Source: CAD feature listing. Evaluate the final solid. Frame: model axes, mm. A direction names the side the tool comes from. Coordinates: 2 decimals unless noted, no trailing zeros. Order: outer loops, then holes, each group sorted by start corner. A loop starts at its lowest first (then second) coordinate and runs counter-clockwise, first axis right, second up. Notation, with made-up numbers: (-12, 51) -> (25, 51) arc R16 cw to (25, 64) -> close; hole circle Ø3 at (38, -38). An arc over 180 degrees is marked (long way). Write item = value, one per line. Start each with the question number.
Item 1: Ray query, line 1 along X through (y, z) = (2.25, 25); line 2 along Z through (x, y) = (12.5, 2.8). Return the intervals inside material, ascending. Write a range as [from, to].
Item 2: Mould query, pull axis X, two halves, no side actions, for faces 3 (the flat face through (-25, 4.5, 14)), 4 (the flat face through (0, 5, 31)), 5 (the cylindrical face through (-14.9, 23.2, 2.5)). Classes: released by +X, released by -X, zero draft, split by the parting line, or undercut.
Item 3: Section query A-A (x = -12.5). Output: boundary loops of the cut face in (y, z), then the cut area to 3 significant figures.
Item 4: Section query B-B (y = 25). Output: boundary loops of the cut face in (x, z).
Item 5: Set-up query: faces 1 (the flat face through (0, 31, 5)), 2 (the flat face through (0, 0, 25)). Return all of +Z, -Z, +X, -X, +Y, -Y with unobstructed straight access to the full face (end or side cutting, diameter ignored); none if empty.
Item 6: Contact query for flat-ended pins moving along their axis: pin 1 (3.5 mm diameter, centred on x = -12.5, z = 25, fed in from -Y); pin 2 (1 mm diameter, centred on x = -1.5, y = 40.5, fed in from +Z); pin 3 (1.5 mm diameter, centred on x = -19.5, z = 17.5, fed in from +Y). Output: stop coordinate, or through.
Item 7: Section query D-D (x = 22.5). Output: boundary loops of the cut face in (y, z).
Autodesk Inventor part; units mm, degrees
ref_plane "YZ Plane" through (0, 0, 0) normal (1, 0, 0) x (0, 1, 0)
ref_plane "XZ Plane" through (0, 0, 0) normal (0, 1, 0) x (-1, 0, 0)
ref_plane "XY Plane" through (0, 0, 0) normal (0, 0, 1) x (1, 0, 0)
sketch "Sketch1" plane through (0, 0, 0) normal (1, 0, 0) x (0, 1, 0)
  line L0 (0, 0) -> (5, 0)
  line L1 (5, 0) -> (5, 50)
  line L2 (5, 50) -> (0, 50)
  line L3 (0, 50) -> (0, 0)
  line L4 (0, 0) -> (50, 0)
  line L5 (50, 0) -> (50, 5)
  line L6 (50, 5) -> (0, 5)
  line L7 (0, 5) -> (0, 0)
  point P0 (5, 5)
  dimension "d0" = 5
  dimension "d1" = 50
  dimension "d2" = 50
  dimension "d3" = 5
extrude "Extrusion1" add sketch "Sketch1" along normal mid plane 50
fillet "Fillet1" radius 7 1 edges at (0, 5, 5)
sketch "Sketch2" plane through (-25, 50, 5) normal (0, 0, 1) x (1, 0, 0)
  line L0 (0, 0) -> (0, -50)
  line L1 (0, 0) -> (0, -25)
  line L2 (12.5, -25) -> (37.5, -25)
  circle A0 centre (12.5, -25) radius 3
  circle A1 centre (37.5, -25) radius 3
  point P0 (25, -50)
  dimension "d7" = 25
  dimension "d8" = 6
  dimension "d9" = 6
sketch "Sketch3" plane through (-25, 5, 50) normal (0, 1, 0) x (1, 0, 0)
  line L0 (0, 50) -> (0, 0)
  line L1 (0, 0) -> (0, 25)
  line L2 (12.5, 25) -> (37.5, 25)
  circle A0 centre (12.5, 25) radius 3
  circle A1 centre (37.5, 25) radius 3
  point P0 (25, 50)
  dimension "d10" = 25
  dimension "d11" = 6
  dimension "d12" = 6
extrude "Extrusion2" cut sketch "Sketch2" against normal blind 50
extrude "Extrusion3" cut sketch "Sketch3" against normal blind 50
properties part number "lclamp"
Computed:
q1.line_1 = [-25, -15.5], [-9.5, 9.5], [15.5, 25]
q1.line_2 = [0, 22], [28, 50]
q2.face_3 = released by -X
q2.face_4 = zero draft
q2.face_5 = undercut
q3.outline = (0, 0) -> (22, 0) -> (22, 5) -> (12, 5) arc R7 cw to (5, 12) -> (5, 22) -> (0, 22) -> close; (0, 28) -> (5, 28) -> (5, 50) -> (0, 50) -> close; (28, 0) -> (50, 0) -> (50, 5) -> (28, 5) -> close
q3.area = 426 mm^2
q4.outline = (-25, 0) -> (-15.5, 0) -> (-15.5, 5) -> (-25, 5) -> close; (-9.5, 0) -> (9.5, 0) -> (9.5, 5) -> (-9.5, 5) -> close; (15.5, 0) -> (25, 0) -> (25, 5) -> (15.5, 5) -> close
q5.face_1 = +Z, +X, -X, +Y
q5.face_2 = +Z, -Z, +X, -X, -Y
q6.pin_1 = through
q6.pin_2 = 5
q6.pin_3 = 5
q7.outline = (0, 0) -> (50, 0) -> (50, 5) -> (12, 5) arc R7 cw to (5, 12) -> (5, 50) -> (0, 50) -> close
